from build123d import *

# Parameters (mm, degrees)
SKETCH2_R           = 3.5
BOSS_EXTRUDE1_DEPTH = 4.5
SKETCH3_OUTSIDE_W   = 21.316
SKETCH3_OUTSIDE_H   = 23.404
SKETCH3_OUTSIDE_W_2 = 8
SKETCH3_OUTSIDE_H_2 = 19.758973988
CUT_EXTRUDE1_DEPTH  = 4.5
CUT_EXTRUDE2_DEPTH  = 1.5


with BuildPart() as part:
    # Sketch1 → Revolve1 (revolve)
    with BuildSketch(Plane.XY, mode=Mode.PRIVATE) as revolve1_sk:
        Polygon((-3.5, 0), (-6.269042262, 0), (-6.5, 9), (-6.5, 20.5), (0, 20.5), (0, 19.5), (-2.5, 18.170968217), (-2.5, 14.885545964), (-3.5, 14.885545964), align=None)
    revolve(revolve1_sk.sketch.rotate(Axis((0, 0, 0), (0, 1, 0)), 180), axis=Axis((0, 0, 0), (0, 1, 0)))

    # Sketch2 → Boss-Extrude1 (add)
    with BuildSketch(Plane(origin=(0, 9, 0), x_dir=(-1, 0, 0), z_dir=(0, -1, 0))):
        Polygon((0, 7.794228634), (-6.75, 3.897114317), (-6.75, -3.897114317), (0, -7.794228634), (6.75, -3.897114317), (6.75, 3.897114317), align=None)
        with Locations(Location((0, 0, 0), (0, 0, 180))):
            Circle(SKETCH2_R, mode=Mode.SUBTRACT)
    extrude(amount=-BOSS_EXTRUDE1_DEPTH)

    # Sketch3 outside → Cut-Extrude1 (cut)
    with BuildSketch(Plane(origin=(0, 20.5, 0), x_dir=(1, 0, 0), z_dir=(0, 1, 0))):
        Rectangle(SKETCH3_OUTSIDE_W, SKETCH3_OUTSIDE_H)
        Rectangle(SKETCH3_OUTSIDE_W_2, SKETCH3_OUTSIDE_H_2, mode=Mode.SUBTRACT)
    extrude(amount=-CUT_EXTRUDE1_DEPTH, mode=Mode.SUBTRACT)

    # Sketch4 → Cut-Extrude2 (cut, symmetric)
    with BuildSketch(Plane(origin=(0, 0, 0), x_dir=(0, 0, -1), z_dir=(1, 0, 0))):
        Polygon((-1.5, 20.5), (1.5, 20.5), (6.937499451, 18.178686883), (6.937499451, 21.048014109), (-6.937499451, 21.048014109), (-6.937499451, 18.178686883), align=None)
    extrude(amount=CUT_EXTRUDE2_DEPTH, both=True, mode=Mode.SUBTRACT)

    # Sketch8 → Cut-Revolve2 (revolve, cut)
    with BuildSketch(Plane.XY):
        with BuildLine():
            Line((-0.75, 19.3), (-0.353553391, 18.903553391))
            ThreePointArc((-0.353553391, 18.903553391), (0, 18.757106781), (0.353553391, 18.903553391))
            Line((0.353553391, 18.903553391), (0.75, 19.3))
            Line((0.75, 19.3), (0.75, 25.5))
            Line((0.75, 25.5), (-0.75, 25.5))
            Line((-0.75, 25.5), (-0.75, 19.3))
        make_face()
    revolve(axis=Axis((0, 25.5, 0), (-1, 0, 0)), mode=Mode.SUBTRACT)


solid = part.part
Source: CAD feature listing. Evaluate the final solid. Frame: model axes, mm. A direction names the side the tool comes from. Round coordinates to 2 decimals unless told otherwise and drop trailing zeros. Order: outer loops, then holes, each group sorted by start corner. A loop starts at its lowest first (then second) coordinate and runs counter-clockwise, first axis right, second up. Notation, with made-up numbers: (15, 5.25) - (33, 5.25) arc R21 ccw to (33, 11.25) - close; hole circle Ø9 at (61, 63.25). An arc over 180 degrees is marked (long way). Use a Markdown table: item, result. Add a question column.
1. Mould query, pull axis X, two halves, no side actions, for faces 6 (the flat face through (-6.75, 11, 0)), 7 (the conical face through (-0.6, 19.2, -0.8)), 8 (the flat face through (-2, 20.5, 0)). Classes: +X half, -X half, draft (parallel to the pull), parting line (faces both ways), or undercut.
2. Section query D-D (y = 1.5). Return the cut outline in (x, z), then the cut area to 3 significant figures.
3. Set-up query: faces 1 (the flat face through (5, 16, 0)), 2 (the flat face through (6, 13.5, 3)), 3 (the flat face through (-1.5, 20, -5)), 4 (the flat face through (1.5, 20, 4)), 5 (the flat face through (-2, 14.886, 2)). Return all of +Z, -Z, +X, -X, +Y, -Y with unobstructed straight access to the full face (end or side cutting, diameter ignored); none if empty.
4. First-contact query: pin 1 (2 mm diameter, centred on x = 0.5, z = 0, fed in from -Y); pin 2 (2.5 mm diameter, centred on y = 19, z = -4.5, fed in from +X); pin 3 (0.6 mm diameter, centred on y = 19.5, z = -3.5, fed in from -X). Flat tips, straight axial feed; report the tip coordinate or a pass-through.
5. Line query: probe 1 along Z at (x, y) = (0, 16.1); probe 2 along Z at (x, y) = (0, 6.75); probe 3 along X at (y, z) = (4, 1.75). Output: solid intervals per line, ascending.
6. Section query A-A (y = 12.5). Return the cut outline in (x, z), then the cut area to 3 significant figures.
7. Section query C-C (y = 7.5). Return the cut outline in (x, z), then the cut area to 3 significant figures.
Derived:
| question | item | result |
|---|---|---|
| 1 | face 6 | -X half |
| 1 | face 7 | undercut |
| 1 | face 8 | draft |
| 2 | outline | circle Ø12.62 at (0, 0); hole circle Ø7 at (0, 0) |
| 2 | area | 86.5 mm2 |
| 3 | face 1 | +Z, -Z, +X, +Y |
| 3 | face 2 | +Y |
| 3 | face 3 | -Z, +Y |
| 3 | face 4 | +Z, +Y |
| 3 | face 5 | -Y |
| 4 | pin 1 | y = 18.7 |
| 4 | pin 2 | x = 4 |
| 4 | pin 3 | x = -4 |
| 5 | probe 1 | -6.5 to -2.5, 2.5 to 6.5 |
| 5 | probe 2 | -6.44 to -3.5, 3.5 to 6.44 |
| 5 | probe 3 | -6.13 to -3.03, 3.03 to 6.13 |
| 6 | outline | (-6.75, -3.9) - (0, -7.79) - (6.75, -3.9) - (6.75, 3.9) - (0, 7.79) - (-6.75, 3.9) - close; hole circle Ø7 at (0, 0) |
| 6 | area | 119 mm2 |
| 7 | outline | circle Ø12.92 at (0, 0); hole circle Ø7 at (0, 0) |
| 7 | area | 92.7 mm2 |
